Design review of the part built by this model. Coordinates are the model's own, in mm. Face numbers are marked on the shaded views. A direction names the side the tool comes from. Coordinates: 2 decimals unless noted, no trailing zeros. Write each loop counter-clockwise with the first axis right and the second up, starting at its lowest first coordinate (ties: lowest second). Pieces come first, ordered by that corner, then holes. Notation, with made-up numbers: (10.5, 12.25) -> (31.5, 12.25) arc R31 cw to (31.5, 45.25) -> close; hole circle Ø7 at (36, 55). An arc over 180 degrees is marked (long way). Write item = value, one per line. Start each with the question number.
```python
from build123d import *

# Parameters (mm, degrees)
F1_DEPTH = 5
F2_R     = 0.5
F3_SIZE  = 1


with BuildPart() as f1:
    # F0 (on Top) → F1 (new body)
    with BuildSketch(Plane.XY):
        with BuildLine():
            ThreePointArc((4.582576, -2), (-5, 0), (4.582576, 2))
            Line((4.582576, 2), (10.41389, 2))
            Line((10.41389, 2), (10.41389, 5))
            Line((10.41389, 5), (8.41389, 5))
            Line((8.41389, 5), (8.41389, 4))
            Line((8.41389, 4), (5.744563, 4))
            ThreePointArc((5.744563, 4), (-7, 0), (5.744563, -4))
            Line((5.744563, -4), (8.41389, -4))
            Line((8.41389, -4), (8.41389, -5))
            Line((8.41389, -5), (10.41389, -5))
            Line((10.41389, -5), (10.41389, -2))
            Line((10.41389, -2), (4.582576, -2))
        make_face()
    extrude(amount=F1_DEPTH)

    # F2
    f2_edges = [f1.edges().sort_by_distance(p)[0] for p in [
        (10.41389, 2, 2.5),
        (4.582576, 2, 2.5),
        (4.582576, -2, 2.5),
        (10.41389, -2, 2.5),
    ]]
    fillet(f2_edges, radius=F2_R)

    # F3
    f3_edges = [f1.edges().sort_by_distance(p)[0] for p in [
        (10.41389, -5, 2.5),
        (10.41389, 5, 2.5),
    ]]
    chamfer(f3_edges, length=F3_SIZE)


solid = f1.part
```
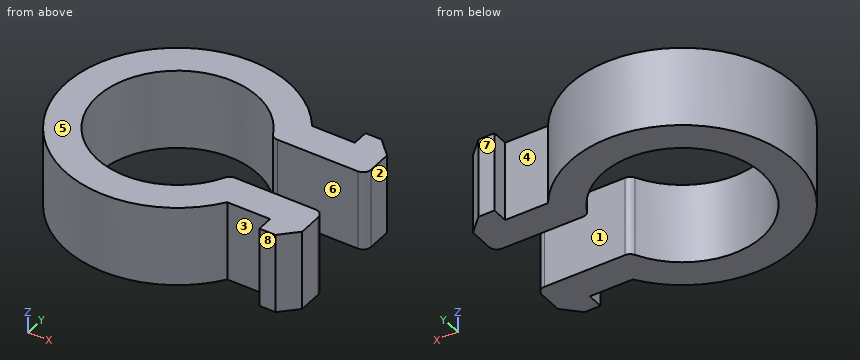
(1) Take a section at C-C, the plane z = 3.65. State the section outline as (x, y) points.
(2) Take a section at D-D, the plane y = 0. State the section outline as (x, z) points, then the cut area to 3 significant figures.
(3) For line 1 (Y direction, x = 0, z = 3.5); line 2 (Y direction, x = 9, z = 4.55); line 3 (X direction, y = 2.75, z = 1.15), list the stretches that pass through material, from the lowest coordinate up.
(4) Take a section at A-A, the plane x = 0. State the section outline as (y, z) points.
(5) Take a section at B-B, the plane y = 3. State the section outline as (x, z) points, then the cut area to 3 significant figures.
(6) For pin 1 Ø0.8 at (y, z) = (4.5, 3) entering from -X; pin 2 Ø1.5 at (x, z) = (7, 2.5) entering from -Y; pin 3 Ø0.5 at (y, z) = (-4.5, 1.5) entering from -X, all flat-tipped, find the tip position at first contact; note any pin that passes through.
(7) For the marked faces 1, 2, 3, 4 and 5, list the 3-axis set-ups (+Z, -Z, +X, -X, +Y, -Y) from which the entire face can be reached by the end or side of a thin tool; tool diameter is ignored.
(8) Mouldability with a two-part tool opening along Y and no side actions: class the marked faces 6, 7 and 8 as pulls with the +Y half, pulls with the -Y half, needs draft (parallel to the pull), parting line crosses it, or undercut.
Report:
q1.outline = (4.45, -2.27) arc R5 cw (long way) to (4.45, 2.27) arc R0.5 ccw to (4.9, 2) -> (9.91, 2) arc R0.5 ccw to (10.41, 2.5) -> (10.41, 4) -> (9.41, 5) -> (8.41, 5) -> (8.41, 4) -> (5.74, 4) arc R7 ccw (long way) to (5.74, -4) -> (8.41, -4) -> (8.41, -5) -> (9.41, -5) -> (10.41, -4) -> (10.41, -2.5) arc R0.5 ccw to (9.91, -2) -> (4.9, -2) arc R0.5 ccw to start
q2.outline = (-7, 0) -> (-5, 0) -> (-5, 5) -> (-7, 5) -> close
q2.area = 10.0 mm2
q3.line_1 = -7 to -5, 5 to 7
q3.line_2 = -5 to -2, 2 to 5
q3.line_3 = -6.44 to -4.18, 4.18 to 10.41
q4.outline = (-7, 0) -> (-5, 0) -> (-5, 5) -> (-7, 5) -> close; (5, 0) -> (7, 0) -> (7, 5) -> (5, 5) -> close
q5.outline = (-6.32, 0) -> (-4, 0) -> (-4, 5) -> (-6.32, 5) -> close; (4, 0) -> (10.41, 0) -> (10.41, 5) -> (4, 5) -> close
q5.area = 43.7 mm2
q6.pin_1 = -5.67
q6.pin_2 = -4
q6.pin_3 = -5.56
q7.face_1 = +Z, -Z, +X
q7.face_2 = +Z, -Z, +X, +Y, -Y
q7.face_3 = +Z, -Z, -Y
q7.face_4 = +Z, -Z, +Y
q7.face_5 = +Z, +X, -X, +Y, -Y
q8.face_6 = undercut
q8.face_7 = pulls with the +Y half
q8.face_8 = pulls with the -Y half
